The model under review builds one solid part; all positions refer to its coordinate system, in mm. A direction names the side the tool comes from. Coordinates: 2 decimals unless noted, no trailing zeros. Write each loop counter-clockwise with the first axis right and the second up, starting at its lowest first coordinate (ties: lowest second). Pieces come first, ordered by that corner, then holes. Notation, with made-up numbers: (-36, -14) - (-5, -14) arc R11 ccw to (-5, 1) - close; hole circle Ø8 at (87.25, 52). An arc over 180 degrees is marked (long way). Return JSON: item names as keys, results as strings. Group by question number.
(1) To check wall thickness, follow L1, parallel to X at y = 14.75, z = 0; L2, parallel to Y at x = 20, z = 16.5. State the ranges of each line that lie inside material, in increasing order. Write a range as from..to.
(2) For pin 1 Ø1 at (y, z) = (14, -7) entering from +X; pin 2 Ø1.5 at (x, z) = (-18, 0) entering from -Y; pin 3 Ø1.5 at (y, z) = (10.5, -10.5) entering from -X; pin 4 Ø6 at (x, y) = (16, 8.5) entering from -Z, all flat-tipped, find the tip position at first contact; note any pin that passes through.
(3) Draft analysis for pull direction X (two halves, no side actions). For faces 1 (the face through (-17, 24, 8)), 2 (the face through (-11.09, 11.83, -14.47)), 3 (the face through (17.38, 13.86, 11.08)), state which applies: released by +X, released by -X, zero draft, split by the parting line, or undercut.
(4) We need section B-B on x = -3. State the section outline as (y, z) points.
(5) We need section C-C on y = 10. State the section outline as (x, z) points, then the cut area to 3 significant figures.
(6) Tool access review of faces 4 (the face through (-13, 0, 13)), 5 (the face through (7, 4, 20)): name each direction out of +Z, -Z, +X, -X, +Y, -Y from which nothing blocks a thin tool from reaching the whole face with its end or side.
(7) We need section A-A on z = 0. State the section outline as (x, y) points.
(8) We need section D-D on x = 23. State the section outline as (y, z) points.
```python
from build123d import *

# Parameters (mm, degrees)
SKETCH1_R           = 30
BOSS_EXTRUDE1_DEPTH = 4
SKETCH1_3_R         = 20.610704172
BOSS_EXTRUDE2_DEPTH = 24
SKETCH1_6_R         = 18.231835924
CUT_EXTRUDE1_DEPTH  = 49.744230428


with BuildPart() as part:
    # Sketch1 → Boss-Extrude1 (new body)
    with BuildSketch(Plane(origin=(0, 0, 0), x_dir=(1, 0, 0), z_dir=(0, 1, 0))):
        with Locations(Location((0, 0, 0), (0, 0, 270))):
            Circle(SKETCH1_R)
    extrude(amount=BOSS_EXTRUDE1_DEPTH)

    # Sketch1_3 → Boss-Extrude2 (add)
    with BuildSketch(Plane(origin=(0, 0, 0), x_dir=(1, 0, 0), z_dir=(0, 1, 0))):
        with Locations(Location((0, 0, 0), (0, 0, 270))):
            Circle(SKETCH1_3_R)
    extrude(amount=BOSS_EXTRUDE2_DEPTH)

    # Sketch1_6 → Cut-Extrude1 (cut, through all)
    with BuildSketch(Plane(origin=(0, 0, 0), x_dir=(1, 0, 0), z_dir=(0, 1, 0))):
        with Locations(Location((0, 0, 0), (0, 0, 270))):
            Circle(SKETCH1_6_R)
    extrude(amount=CUT_EXTRUDE1_DEPTH, mode=Mode.SUBTRACT)


solid = part.part
```
Ans:
{
 "1": {"L1": "-20.61..-18.23, 18.23..20.61", "L2": "0..4"},
 "2": {"pin 1": "x = 19.56", "pin 2": "y = 0", "pin 3": "x = -18.16", "pin 4": "z = -15.99"},
 "3": {"face 1": "zero draft", "face 2": "undercut", "face 3": "split by the parting line"},
 "4": {"outline": "(0, -29.85) - (4, -29.85) - (4, -20.39) - (24, -20.39) - (24, -17.98) - (0, -17.98) - close; (0, 17.98) - (24, 17.98) - (24, 20.39) - (4, 20.39) - (4, 29.85) - (0, 29.85) - close"},
 "5": {"outline": "circle Ø41.22 at (0, 0); hole circle Ø36.46 at (0, 0)", "area": "290 mm²"},
 "6": {"face 4": "+Z, -Z, +X, -X, -Y", "face 5": "+Y"},
 "7": {"outline": "(-30, 0) - (-18.23, 0) - (-18.23, 24) - (-20.61, 24) - (-20.61, 4) - (-30, 4) - close; (18.23, 0) - (30, 0) - (30, 4) - (20.61, 4) - (20.61, 24) - (18.23, 24) - close"},
 "8": {"outline": "(0, -19.26) - (4, -19.26) - (4, 19.26) - (0, 19.26) - close"}
}
